Work out the finished part from the listing and answer in its coordinate system (mm). Face numbers are marked on the shaded views. A direction names the side the tool comes from. Give positions to 0.01 mm unless a question says otherwise; leave off trailing zeros. Order: outer loops, then holes, each group sorted by start corner. A loop starts at its lowest first (then second) coordinate and runs counter-clockwise, first axis right, second up. Notation, with made-up numbers: M 40.25,22.5 L 80.25,22.5 A21 ccw 80.25,26.5 Z; hole C 4.25,-39.5 d11. An arc over 180 degrees is marked long. One line per item, written item: value.
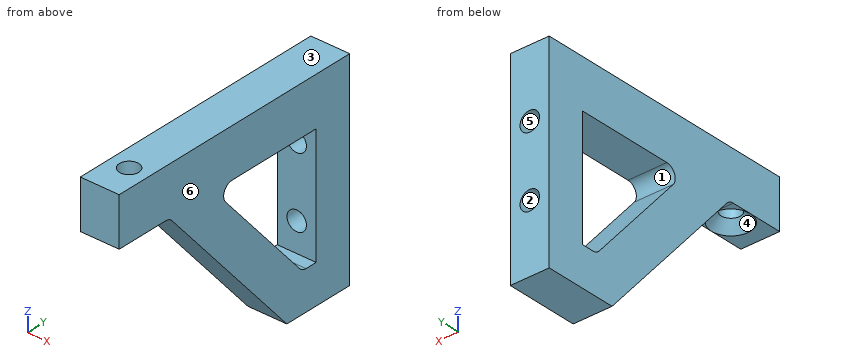
from build123d import *

# Parameters (mm, degrees)
EXTRUDE_1_DEPTH     = 4
CUT_EXTRUDE_1_REACH = 71.622
SKETCH_2_R          = 2
CUT_EXTRUDE_3_REACH = 66.01
SKETCH_4_R          = 2
FILLET_1_R          = 2
CHAMFER_1_SIZE      = 2


with BuildPart() as part:
    # 草图1 → 凸台-拉伸1 (new, symmetric)
    with BuildSketch(Plane(origin=(0, 0, 0), x_dir=(0, 0, -1), z_dir=(1, 0, 0))):
        Polygon((0, 0), (42.5, 0), (42.5, -15), (10, -43), (10, -55), (0, -55), align=None)
        Polygon((10, -32.440459038), (34.5, -11.33276673), (34.5, -8), (10, -8), align=None, mode=Mode.SUBTRACT)
    extrude(amount=EXTRUDE_1_DEPTH, both=True)

    # 草图2 → 切除-拉伸1 (cut, up to next)
    with BuildSketch(Plane(origin=(0, 0, 0), x_dir=(1, 0, 0), z_dir=(0, 1, 0)), mode=Mode.PRIVATE) as cut_extrude_1_sk1:
        with Locations(Location((0, 14, 0), (0, 0, 270))):
            Circle(SKETCH_2_R)
    cut_extrude_1_tool1 = extrude(cut_extrude_1_sk1.sketch, amount=-CUT_EXTRUDE_1_REACH, mode=Mode.PRIVATE) & part.part
    # 草图2 → 切除-拉伸1 (cut, up to next)
    with BuildSketch(Plane(origin=(0, 0, 0), x_dir=(1, 0, 0), z_dir=(0, 1, 0)), mode=Mode.PRIVATE) as cut_extrude_1_sk2:
        with Locations(Location((0, 28.5, 0), (0, 0, 270))):
            Circle(SKETCH_2_R)
    cut_extrude_1_tool2 = extrude(cut_extrude_1_sk2.sketch, amount=-CUT_EXTRUDE_1_REACH, mode=Mode.PRIVATE) & part.part
    add(cut_extrude_1_tool1.solids().sort_by_distance((0, 0, -14))[0], mode=Mode.SUBTRACT)
    add(cut_extrude_1_tool2.solids().sort_by_distance((0, 0, -28.5))[0], mode=Mode.SUBTRACT)

    # 草图4 → 切除-拉伸3 (cut, up to next)
    with BuildSketch(Plane(origin=(0, 0, -10), x_dir=(-1, 0, 0), z_dir=(0, 0, -1)), mode=Mode.PRIVATE) as cut_extrude_3_sk1:
        with Locations(Location((0, -48, 0), (0, 0, 90))):
            Circle(SKETCH_4_R)
    cut_extrude_3_tool1 = extrude(cut_extrude_3_sk1.sketch, amount=-CUT_EXTRUDE_3_REACH, mode=Mode.PRIVATE) & part.part
    add(cut_extrude_3_tool1.solids().sort_by_distance((0, -48, -10))[0], mode=Mode.SUBTRACT)

    # 圆角1
    fillet_1_edges = [part.edges().sort_by_distance(p)[0] for p in [
        (0, -43, -10),
        (0, -32.440459038, -10),
        (0, -11.33276673, -34.5),
    ]]
    fillet(fillet_1_edges, radius=FILLET_1_R)

    # 倒角1
    chamfer_1_edges = [part.edges().sort_by_distance(p)[0] for p in [
        (0, -50, -10),
    ]]
    chamfer(chamfer_1_edges, length=CHAMFER_1_SIZE - 0.0001)  # a hair under: the kernel refuses the full size


solid = part.part
(1) Determine the mould class of the marked faces 4, 5 and 6 for opening direction Z: pulls with the +Z half, pulls with the -Z half, needs draft (parallel to the pull), parting line crosses it, or undercut.
Findings:
face 4: pulls with the -Z half
face 5: undercut
face 6: needs draft
(2) Section C-C, the plane y = -7 is taken. Give the vertices of the cut face in (x, z), then the cut area to 3 significant figures.
Findings:
outline: M -4,-42.5 L 4,-42.5 L 4,0 L -4,0 Z; hole C 0,-28.5 d4; hole C 0,-14 d4
area: 315 mm^2
(3) Section A-A, the plane z = -20 is taken. Give the vertices of the cut face in (x, y), then the cut area to 3 significant figures.
Findings:
outline: M -4,-34.38 L 4,-34.38 L 4,-23.83 L -4,-23.83 Z; M -4,-8 L 4,-8 L 4,0 L -4,0 Z
area: 148 mm^2
(4) Find the intervals of material crossed by probe 1 along X at (y, z) = (-48, -4); probe 2 along Z at (x, y) = (1.25, -16.5); probe 3 along Y at (x, z) = (-2.5, -33), in increasing order. Write a range as from..to.
Findings:
probe 1: x = -4..-2, 2..4
probe 2: z = -40.76..-28.5, -10..0
probe 3: y = -23.18..-12.63, -8..0
(5) Given P1, Ø3, axis at x = -1.5, z = -26.5, coming from the -Y side; P2, Ø3.5, axis at x = 0, z = -28.5, coming from the +Y side; P3, Ø12, axis at y = -37, z = -30, coming from the -X side; P4, Ø3.5, axis at x = 0, z = -14, coming from the -Y side, each flat-ended and moving along its own axis, determine where each tip first touches the part or whether it passes through.
Findings:
P1: stops at y = -30.08
P2: stops at y = -14.99
P3: passes through
P4: stops at y = -41.06
(6) Section D-D, the plane z = -14 is taken. Give the vertices of the cut face in (x, y), then the cut area to 3 significant figures.
Findings:
outline: M -4,-39.55 L 4,-39.55 L 4,-28.99 L -4,-28.99 Z; M -4,-8 L -2,-8 L -2,0 L -4,0 Z; M 2,-8 L 4,-8 L 4,0 L 2,0 Z
area: 116 mm^2
(7) Which of the six approach directions +Z, -Z, +X, -X, +Y, -Y give full straight-line access (tool end or side, diameter ignored) to the marked faces 1, 2 and 3?
Findings:
face 1: +X, -X
face 2: +Y
face 3: +Z, +X, -X, +Y, -Y
